```python
from build123d import *

# Parameters (mm, degrees)
SKETCH1_R           = 1.59
BOSS_EXTRUDE1_DEPTH = 5.2
SKETCH1_5_R         = 1.59
CUT_EXTRUDE2_DEPTH  = 4.2


with BuildPart() as part:
    # Sketch1 → Boss-Extrude1 (new body)
    with BuildSketch(Plane(origin=(0, 0, 0), x_dir=(1, 0, 0), z_dir=(0, 1, 0))):
        Polygon((34.02, 14.134213562), (36.56, 11.594213562), (36.56, -22.004213562), (34.02, -24.544213562), (34.02, -27.67), (-34.02, -27.67), (-34.02, 27.67), (34.02, 27.67), align=None)
        with Locations((33.02, -19.05)):
            Circle(SKETCH1_R, mode=Mode.SUBTRACT)
        with Locations((33.02, 8.89)):
            Circle(SKETCH1_R, mode=Mode.SUBTRACT)
        with Locations((-17.78, 24.13)):
            Circle(SKETCH1_R, mode=Mode.SUBTRACT)
        with Locations((-19.05, -24.13)):
            Circle(SKETCH1_R, mode=Mode.SUBTRACT)
    extrude(amount=-BOSS_EXTRUDE1_DEPTH)

    # Sketch1_5 → Cut-Extrude2 (cut)
    with BuildSketch(Plane(origin=(0, 0, 0), x_dir=(1, 0, 0), z_dir=(0, 1, 0))):
        Polygon((33.02, 13.72), (35.56, 11.18), (35.56, -21.59), (33.02, -24.13), (33.02, -26.67), (-33.02, -26.67), (-33.02, 26.67), (33.02, 26.67), align=None)
        with Locations((-19.05, -24.13)):
            Circle(SKETCH1_5_R, mode=Mode.SUBTRACT)
        with Locations((-17.78, 24.13)):
            Circle(SKETCH1_5_R, mode=Mode.SUBTRACT)
        with Locations((33.02, 8.89)):
            Circle(SKETCH1_5_R, mode=Mode.SUBTRACT)
        with Locations((33.02, -19.05)):
            Circle(SKETCH1_5_R, mode=Mode.SUBTRACT)
    extrude(amount=-CUT_EXTRUDE2_DEPTH, mode=Mode.SUBTRACT)


solid = part.part
```
The listing builds one solid part. Answer for the finished solid, in the listing's coordinates (mm). A direction names the side the tool comes from. Give positions to 0.01 mm unless a question says otherwise; leave off trailing zeros. Order: outer loops, then holes, each group sorted by start corner. A loop starts at its lowest first (then second) coordinate and runs counter-clockwise, first axis right, second up. Notation, with made-up numbers: (40, -4.75) -> (80, -4.75) arc R25 ccw to (80, 26.25) -> close; hole circle Ø2 at (4.25, 41.5). An arc over 180 degrees is marked (long way). Write each question's results on one line, items separated by ' | '.
Q1. Straight lines are drawn through the part: probe 1 along Z at (x, y) = (33.02, -4.6); probe 2 along Z at (x, y) = (1.5, -3.15); probe 3 along Z at (x, y) = (-17.78, -4.45). For each, find the intervals that lie inside material, in ascending order. Write a range as from..to.
Checked values:
probe 1: z = -27.67..-10.48, -7.3..17.46, 20.64..27.67 | probe 2: z = -27.67..-26.67, 26.67..27.67 | probe 3: z = -27.67..-25.72, -22.54..23.17, 25.09..27.67
Q2. Determine the mould class of faces 1 (the face through (1, 0, -27)), 2 (the face through (-34.02, -3, 0)), 3 (the face through (-17.987, -4.693, -25.706)), 4 (the face through (0, -2, -26.67)) for opening direction X: pulls with the +X half, pulls with the -X half, needs draft (parallel to the pull), parting line crosses it, or undercut.
Checked values:
face 1: needs draft | face 2: pulls with the -X half | face 3: undercut | face 4: undercut
Q3. The part is cut by section B-B, the plane x = 14.5. Give the vertices of the cut face in (y, z), and give its area (3 significant figures).
Checked values:
outline: (-5.2, -27.67) -> (0, -27.67) -> (0, -26.67) -> (-4.2, -26.67) -> (-4.2, 26.67) -> (0, 26.67) -> (0, 27.67) -> (-5.2, 27.67) -> close | area: 63.7 mm^2
Q4. The part is cut by section A-A, the plane z = 19.05. Give the vertices of the cut face in (x, y).
Checked values:
outline: (-34.02, -5.2) -> (31.43, -5.2) -> (31.43, -4.2) -> (-33.02, -4.2) -> (-33.02, 0) -> (-34.02, 0) -> close; (34.61, -5.2) -> (36.56, -5.2) -> (36.56, 0) -> (35.56, 0) -> (35.56, -4.2) -> (34.61, -4.2) -> close
Q5. Which of the six approach directions +Z, -Z, +X, -X, +Y, -Y give full straight-line access (tool end or side, diameter ignored) to faces 5 (the face through (34.02, -3, 26)), 6 (the face through (0, -2, 26.67)), 7 (the face through (34.02, -3, -21))?
Checked values:
face 5: +Z, +X, +Y, -Y | face 6: +Y | face 7: -Z, +X, +Y, -Y
Q6. The part is cut by section C-C, the plane z = -1.5. Give the vertices of the cut face in (x, y).
Checked values:
outline: (-34.02, -5.2) -> (36.56, -5.2) -> (36.56, 0) -> (35.56, 0) -> (35.56, -4.2) -> (-33.02, -4.2) -> (-33.02, 0) -> (-34.02, 0) -> close
Q7. The part is cut by section D-D, the plane z = -24.13. Give the vertices of the cut face in (x, y), and give its area (3 significant figures).
Checked values:
outline: (-34.02, -5.2) -> (-19.37, -5.2) -> (-19.37, -4.2) -> (-33.02, -4.2) -> (-33.02, 0) -> (-34.02, 0) -> close; (-16.19, -5.2) -> (34.02, -5.2) -> (34.02, 0) -> (33.02, 0) -> (33.02, -4.2) -> (-16.19, -4.2) -> close | area: 73.3 mm^2
Q8. Each of these flat-tipped pins is pushed along its axis until it touches: P1, Ø4, axis at x = 33.02, z = -8.89, coming from the +Y side; P2, Ø3, axis at x = -17.78, z = -24.13, coming from the -Y side; P3, Ø2.5, axis at y = -2, z = -19.5, coming from the +X side; P4, Ø2.5, axis at y = -2, z = 25.5, coming from the +X side. Where does it stop, or does it pass through?
Checked values:
P1: stops at y = -4.2 | P2: passes through | P3: stops at x = 34.02 | P4: stops at x = 34.31
